Check sheet for the modelled part. Datum: model origin and axes. Units: mm. Give positions to 0.01 mm unless a question says otherwise; leave off trailing zeros. Write each loop counter-clockwise with the first axis right and the second up, starting at its lowest first coordinate (ties: lowest second). Pieces come first, ordered by that corner, then holes. Notation, with made-up numbers: (-2.5, -3) -> (36.5, -3) arc R32 cw to (36.5, 25) -> close; hole circle Ø8 at (19, -4.75). An arc over 180 degrees is marked (long way). Return JSON: item names as keys, results as strings.
from build123d import *

# Parameters (mm, degrees)
SKETCH1_W                       = 50.8
SKETCH1_H                       = 50.8
SKETCH1_R                       = 14.2748
BOSS_EXTRUDE1_DEPTH             = 3.175
FILLET1_R                       = 2.54
F_5_32_0_15625_DIAMETER_HOLE1_D = 3.96875


with BuildPart() as part:
    # Sketch1 → Boss-Extrude1 (new body)
    with BuildSketch(Plane.XY):
        Rectangle(SKETCH1_W, SKETCH1_H)
        Circle(SKETCH1_R, mode=Mode.SUBTRACT)
    extrude(amount=BOSS_EXTRUDE1_DEPTH)

    # Fillet1
    fillet1_edges = [part.edges().sort_by_distance(p)[0] for p in [
        (-25.4, 25.4, 1.5875),
        (25.4, 25.4, 1.5875),
        (25.4, -25.4, 1.5875),
        (-25.4, -25.4, 1.5875),
    ]]
    fillet(fillet1_edges, radius=FILLET1_R)

    # 5/32 (0.15625) Diameter Hole1 (through all)
    with Locations(Plane.XY.offset(3.175)):
        with Locations((-19.05, 19.05), (19.05, 19.05), (19.05, -19.05), (-19.05, -19.05)):
            Hole(F_5_32_0_15625_DIAMETER_HOLE1_D / 2)


solid = part.part
(1) Cross-section at A-A on x = -19.05. Enter the section's corners in (y, z) (3 decimals).
Reply:
{"outline": "(-25.4, 0) -> (-21.034, 0) -> (-21.034, 3.175) -> (-25.4, 3.175) -> close; (-17.066, 0) -> (17.066, 0) -> (17.066, 3.175) -> (-17.066, 3.175) -> close; (21.034, 0) -> (25.4, 0) -> (25.4, 3.175) -> (21.034, 3.175) -> close"}
(2) Thickness scan on L1, parallel to Y at x = -19, z = 1.1; L2, parallel to Y at x = 0, z = 2.05; L3, parallel to Y at x = -20, z = 2.5. Record the ranges inside material, lowest first.
Reply:
{"L1": "-25.4 to -21.03, -17.07 to 17.07, 21.03 to 25.4", "L2": "-25.4 to -14.27, 14.27 to 25.4", "L3": "-25.4 to -20.79, -17.31 to 17.31, 20.79 to 25.4"}
(3) Depth check by flat-ended pin: pin 1 Ø17 at (x, y) = (0, 0) entering from -Z. Enter the tip coordinate at first touch or a pass-through.
Reply:
{"pin 1": "through"}
(4) Release check for a two-part mould opening along X. For faces 1 (the flat face through (11, -11, 0)), 2 (the cylindrical face through (-18.62, -20.987, 1.565)), 3 (the flat face through (-25.4, 0, 2)) record: pulls with the +X half, pulls with the -X half, needs draft (parallel to the pull), parting line crosses it, or undercut.
Reply:
{"face 1": "needs draft", "face 2": "undercut", "face 3": "pulls with the -X half"}
(5) Cross-section at C-C on z = 0.7. Enter the section's corners in (x, y), then the cut area to 3 significant figures.
Reply:
{"outline": "(-25.4, -22.86) arc R2.54 ccw to (-22.86, -25.4) -> (22.86, -25.4) arc R2.54 ccw to (25.4, -22.86) -> (25.4, 22.86) arc R2.54 ccw to (22.86, 25.4) -> (-22.86, 25.4) arc R2.54 ccw to (-25.4, 22.86) -> close; hole circle Ø3.97 at (-19.05, -19.05); hole circle Ø3.97 at (-19.05, 19.05); hole circle Ø28.55 at (0, 0); hole circle Ø3.97 at (19.05, -19.05); hole circle Ø3.97 at (19.05, 19.05)", "area": "1,890 mm^2"}
(6) Cross-section at B-B on y = 0. Enter the section's corners in (x, z) (3 decimals), then the cut area to 3 significant figures.
Reply:
{"outline": "(-25.4, 0) -> (-14.275, 0) -> (-14.275, 3.175) -> (-25.4, 3.175) -> close; (14.275, 0) -> (25.4, 0) -> (25.4, 3.175) -> (14.275, 3.175) -> close", "area": "70.6 mm^2"}
